Verification items for the finished model (mm, model axes). A direction names the side the tool comes from. Coordinates: 2 decimals unless noted, no trailing zeros. Write each loop counter-clockwise with the first axis right and the second up, starting at its lowest first coordinate (ties: lowest second). Pieces come first, ordered by that corner, then holes. Notation, with made-up numbers: (53, 29) -> (110, 29) arc R9 cw to (110, 34) -> close; hole circle Ø3 at (-35.5, 80.5). An arc over 180 degrees is marked (long way). Answer in a Markdown table with one row per item.
```python
from build123d import *

# Parameters (mm, degrees)
BOSS_EXTRUDE1_DEPTH                   = 3.5
CUT_EXTRUDE1_DEPTH                    = 39.124532784
TAP_DRILL_FOR_M2X0_4_TAP1_D           = 1.6
TAP_DRILL_FOR_M2X0_4_TAP1_ON_FACE_2_D = 1.6


with BuildPart() as part:
    # Sketch1 → Boss-Extrude1 (new, symmetric)
    with BuildSketch(Plane(origin=(0, 0, 0), x_dir=(1, 0, 0), z_dir=(0, 1, 0))):
        with BuildLine():
            Line((-19.499743588, -0.1), (-26.49981132, -0.1))
            ThreePointArc((-26.49981132, -0.1), (-18.738329701, -18.738329701), (-0.1, -26.49981132))
            Line((-0.1, -26.49981132), (-0.1, -19.499743588))
            ThreePointArc((-0.1, -19.499743588), (-13.788582233, -13.788582233), (-19.499743588, -0.1))
        make_face()
    extrude(amount=BOSS_EXTRUDE1_DEPTH, both=True)

    # Sketch2 → Cut-Extrude1 (cut, through all)
    with BuildSketch(Plane(origin=(0, 3.5, 0), x_dir=(1, 0, 0), z_dir=(0, 1, 0))):
        Polygon((-22.273863607, -15.202795796), (-15.202795796, -22.273863607), (-12.02081528, -19.091883092), (-19.091883092, -12.02081528), align=None)
    extrude(amount=-CUT_EXTRUDE1_DEPTH, mode=Mode.SUBTRACT)

    # Tap Drill for M2x0.4 Tap1 (through all)
    with Locations(Plane(origin=(-17.324116139, 0, 13.788582233), x_dir=(0.707106781187, 0, 0.707106781187), z_dir=(-0.707106781187, 0, 0.707106781187))):
        with Locations((0, 0)):
            Hole(TAP_DRILL_FOR_M2X0_4_TAP1_D / 2)

    # Tap Drill for M2x0.4 Tap1 on face 2 (through all)
    with Locations(Plane(origin=(-13.788582233, 0, 17.324116139), x_dir=(0.707106781187, 0, 0.707106781187), z_dir=(-0.707106781187, 0, 0.707106781187))):
        with Locations((0, 0)):
            Hole(TAP_DRILL_FOR_M2X0_4_TAP1_ON_FACE_2_D / 2)


solid = part.part
```
1. Thickness scan on line 1 (X direction, y = 0, z = 13); line 2 (Z direction, x = -21, y = 1.5); line 3 (Z direction, x = -24.5, y = 0). Record the ranges inside material, lowest first. Write a range as from..to.
Geometry says:
| item | result |
|---|---|
| line 1 | -23.09..-20.07, -18.11..-17.67, -15.4..-14.53 |
| line 2 | 0.1..13.93 |
| line 3 | 0.1..10.1 |
2. Tool access check on faces 1 (the flat face through (-20.49, 0.05, 13.42)), 2 (the flat face through (-23, 0, 0.1)), 3 (the flat face through (-15.507, 0.049, 15.606)), 4 (the flat face through (-13.46, 0.05, 20.53)). Record the directions out of +Z, -Z, +X, -X, +Y, -Y that give a thin tool (end or side, any length) a straight path to the whole face; none if there is none.
Geometry says:
| item | result |
|---|---|
| face 1 | +Z, +Y, -Y |
| face 2 | -Z, +X, -X, +Y, -Y |
| face 3 | +Y, -Y |
| face 4 | -X, +Y, -Y |
3. Section check C-C, the plane z = 4.5. Record the boundary of the cut face in (x, y).
Geometry says:
| item | result |
|---|---|
| outline | (-26.12, -3.5) -> (-18.97, -3.5) -> (-18.97, 3.5) -> (-26.12, 3.5) -> close |
4. Section check A-A, the plane y = -1.5. Record the boundary of the cut face in (x, z), plus the area to 3 significant figures.
Geometry says:
| item | result |
|---|---|
| outline | (-26.5, 0.1) -> (-19.5, 0.1) arc R19.5 cw to (-0.1, 19.5) -> (-0.1, 26.5) arc R26.5 ccw to (-14.87, 21.94) -> (-12.02, 19.09) -> (-19.09, 12.02) -> (-21.94, 14.87) arc R26.5 ccw to start |
| area | 208 mm^2 |
5. Section check B-B, the plane x = -8.5. Record the boundary of the cut face in (y, z).
Geometry says:
| item | result |
|---|---|
| outline | (-3.5, 17.55) -> (3.5, 17.55) -> (3.5, 25.1) -> (-3.5, 25.1) -> close |
6. Depth check by flat-ended pin: P1, Ø2, axis at x = -4.5, y = -1.5, coming from the -Z side; P2, Ø4, axis at x = -3, y = 1.5, coming from the +Z side; P3, Ø3, axis at y = -2, z = 18.5, coming from the -X side. Enter the tip coordinate at first touch or a pass-through.
Geometry says:
| item | result |
|---|---|
| P1 | z = 18.71 |
| P2 | z = 26.48 |
| P3 | x = -14.11 |
7. Mould release check, pull along Z, two halves, no side actions. Record for faces 5 (the cylindrical face through (-7.928, 0.049, 25.286)), 6 (the flat face through (-0.1, 0, 23)), 7 (the cylindrical face through (-13.637, 0.049, 13.938)), 8 (the cylindrical face through (-12.226, 0.035, 16.892)): released by +Z, released by -Z, zero draft, split by the parting line, or undercut.
Geometry says:
| item | result |
|---|---|
| face 5 | released by +Z |
| face 6 | zero draft |
| face 7 | released by -Z |
| face 8 | undercut |
